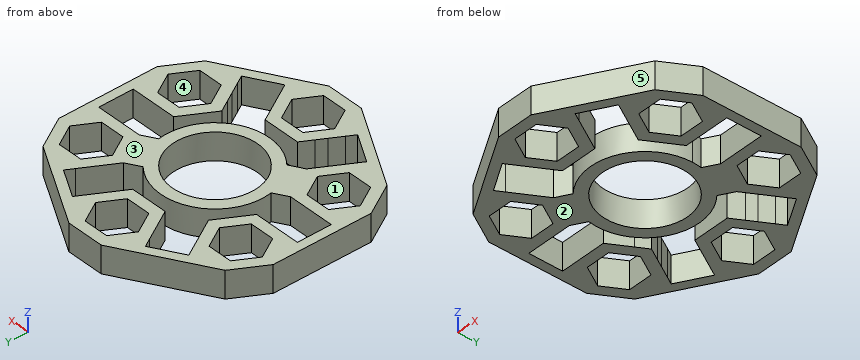
from build123d import *

# Parameters (mm, degrees)
F0_R     = 11.0786603321
F0_R_2   = 10.9474
F1_DEPTH = 6.9977
F2_R     = 13.2854455685
F2_R_2   = 11.176
F3_DEPTH = 6.9977


# Not quite as in the source:
# - a feature names something its author has since deleted; it is built from what else it names


with BuildPart() as f1:
    # F0 (on Top) → F1 (new body)
    with BuildSketch(Plane.XY):
        with BuildLine():
            ThreePointArc((8.9895158912, 10.693432753), (-6.985, 12.0983748909), (-13.7555423633, -2.438432753))
            ThreePointArc((-13.7555423633, -2.438432753), (-12.0983748909, -6.985), (-8.9895158912, -10.693432753))
            ThreePointArc((-8.9895158912, -10.693432753), (5.8981930708, -12.6638153216), (13.97, 0))
            ThreePointArc((13.97, 0), (13.9162823127, 1.2239226251), (13.7555423633, 2.438432753))
            ThreePointArc((13.7555423633, 2.438432753), (13.347336888, 4.1242572662), (12.7333664349, 5.7465014779))
            ThreePointArc((12.7333664349, 5.7465014779), (11.139521372, 8.4304189458), (8.9895158912, 10.693432753))
        make_face()
        Circle(F0_R, mode=Mode.SUBTRACT)
        Circle(F0_R)
        Circle(F0_R_2, mode=Mode.SUBTRACT)
        Polygon((-14.0807527651, 9.595996083), (-12.3768237899, 12.5472876405), (-14.2130055479, 15.7276477372), (-15.394837026, 17.7746399033), (-17.1428502621, 20.8022876405), (-21.9088767342, 20.8022876405), (-26.6749032064, 20.8022876405), (-31.4409296786, 12.5472876405), (-29.1460849644, 8.5725), (-26.6749032064, 4.2922876405), (-17.1428502621, 4.2922876405), (-15.3507527651, 7.3962915574), align=None)
        Polygon((-18.7559669142, 18.0082876405), (-15.6030570942, 12.5472876405), (-18.7559669142, 7.0862876405), (-25.0617865543, 7.0862876405), (-28.2146963743, 12.5472876405), (-25.0617865543, 18.0082876405), align=None, mode=Mode.SUBTRACT)
        Polygon((4.854194994, 33.5022876405), (-4.6778579503, 33.5022876405), (-7.0608711864, 29.3747876405), (-9.4438844224, 25.2472876405), (-4.6778579503, 16.9922876405), (-1.27, 16.9922876405), (1.27, 16.9922876405), (4.854194994, 16.9922876405), (6.6462924911, 20.0962915574), (7.9162924911, 22.295996083), (9.6202214662, 25.2472876405), (7.2372082301, 29.3747876405), align=None)
        Polygon((6.393988162, 25.2472876405), (3.2410783419, 19.7862876405), (-3.0647412982, 19.7862876405), (-6.2176511182, 25.2472876405), (-3.0647412982, 30.7082876405), (3.2410783419, 30.7082876405), align=None, mode=Mode.SUBTRACT)
        Polygon((-29.1460849644, -8.5725), (-31.5290982004, -12.7), (-26.7630717283, -20.955), (-21.9970452561, -20.955), (-17.231018784, -20.955), (-12.4649923118, -12.7), (-14.2130055479, -9.6723522628), (-15.4830055479, -7.4726477372), (-17.231018784, -4.445), (-20.7270452561, -4.445), (-23.2670452561, -4.445), (-26.7630717283, -4.445), align=None)
        Polygon((-25.150604473, -7.2393749809), (-18.8447848775, -7.2386250963), (-15.6912256606, -12.6992501153), (-18.8434860392, -18.1606250191), (-25.1493056347, -18.1613749037), (-28.3028648516, -12.7007498847), align=None, mode=Mode.SUBTRACT)
        Polygon((31.5290982004, 12.7), (26.7630717283, 20.955), (21.9970452561, 20.955), (17.231018784, 20.955), (12.4649923118, 12.7), (14.2130055479, 9.6723522628), (15.4830055479, 7.4726477372), (17.231018784, 4.445), (20.7270452561, 4.445), (23.2670452561, 4.445), (26.7630717283, 4.445), (29.1460849644, 8.5725), align=None)
        Polygon((25.1499550762, 7.239), (18.8441354361, 7.239), (15.691225616, 12.7), (18.8441354361, 18.161), (25.1499550762, 18.161), (28.3028648962, 12.7), align=None, mode=Mode.SUBTRACT)
        Polygon((-7.1490397082, -29.5275), (-4.7660264722, -33.655), (4.7660264722, -33.655), (7.1490397082, -29.5275), (9.5320529443, -25.4), (4.7660264722, -17.145), (1.27, -17.145), (-1.27, -17.145), (-4.7660264722, -17.145), (-6.5140397082, -20.1726477372), (-7.7840397082, -22.3723522628), (-9.5320529443, -25.4), align=None)
        Polygon((-6.3058196401, -25.4), (-3.15290982, -19.939), (3.15290982, -19.939), (6.3058196401, -25.4), (3.15290982, -30.861), (-3.15290982, -30.861), align=None, mode=Mode.SUBTRACT)
        Polygon((26.7630717283, -20.955), (31.5290982004, -12.7), (29.1460849644, -8.5725), (26.7630717283, -4.445), (17.231018784, -4.445), (12.4649923118, -12.7), (14.2130055479, -15.7276477372), (15.4830055479, -17.9273522628), (17.231018784, -20.955), (21.9970452561, -20.955), align=None)
        Polygon((18.8441354361, -18.161), (15.691225616, -12.7), (18.8441354361, -7.239), (25.1499550762, -7.239), (28.3028648962, -12.7), (25.1499550762, -18.161), align=None, mode=Mode.SUBTRACT)
        Polygon((-26.6749032064, 20.8022876405), (-21.9088767342, 20.8022876405), (-18.3343568801, 22.8660376405), (-10.6353910405, 27.3110376405), (-7.0608711864, 29.3747876405), (-4.6778579503, 33.5022876405), align=None)
        Polygon((-21.9970452561, -20.955), (-26.7630717283, -20.955), (-4.7660264722, -33.655), (-7.1490397082, -29.5275), (-10.7235595624, -27.46375), (-18.422525402, -23.01875), align=None)
        Polygon((31.5290982004, -12.7), (31.5290982004, 12.7), (29.1460849644, 8.5725), (29.1460849644, 4.445), (29.1460849644, -4.445), (29.1460849644, -8.5725), align=None)
        Polygon((7.1490397082, -29.5275), (4.7660264722, -33.655), (26.7630717283, -20.955), (21.9970452561, -20.955), (18.422525402, -23.01875), (10.7235595624, -27.46375), align=None)
        Polygon((26.7630717283, 20.955), (4.854194994, 33.5022876405), (7.2372082301, 29.3747876405), (10.811599772, 27.3357666355), (18.4011736203, 23.0062743808), (21.9970452561, 20.955), align=None)
        Polygon((-29.1460849644, 4.2922876405), (-29.1460849644, 8.5725), (-31.4409296786, 12.5472876405), (-31.5290982004, -12.7), (-29.1460849644, -8.5725), (-29.1460849644, -4.445), align=None)
        with BuildLine():
            Line((-13.7555423633, -2.438432753), (-17.231018784, -4.445))
            Line((-17.231018784, -4.445), (-15.4830055479, -7.4726477372))
            Line((-15.4830055479, -7.4726477372), (-14.2130055479, -9.6723522628))
            Line((-14.2130055479, -9.6723522628), (-12.4649923118, -12.7))
            Line((-12.4649923118, -12.7), (-8.9895158912, -10.693432753))
            ThreePointArc((-8.9895158912, -10.693432753), (-12.0983748909, -6.985), (-13.7555423633, -2.438432753))
        make_face()
        with BuildLine():
            Line((14.2130055479, 9.6723522628), (12.4649923118, 12.7))
            Line((12.4649923118, 12.7), (8.9895158912, 10.693432753))
            ThreePointArc((8.9895158912, 10.693432753), (11.139521372, 8.4304189458), (12.7333664349, 5.7465014779))
            ThreePointArc((12.7333664349, 5.7465014779), (13.347336888, 4.1242572662), (13.7555423633, 2.438432753))
            Line((13.7555423633, 2.438432753), (17.231018784, 4.445))
            Line((17.231018784, 4.445), (15.4830055479, 7.4726477372))
            Line((15.4830055479, 7.4726477372), (14.2130055479, 9.6723522628))
        make_face()
        Polygon((-29.1460849644, 4.2922876405), (-26.6749032064, 4.2922876405), (-29.1460849644, 8.5725), align=None)
        Polygon((10.811599772, 27.3357666355), (7.2372082301, 29.3747876405), (9.6202214662, 25.2472876405), align=None)
        Polygon((-21.9088767342, 20.8022876405), (-17.1428502621, 20.8022876405), (-18.3343568801, 22.8660376405), align=None)
        Polygon((-7.0608711864, 29.3747876405), (-10.6353910405, 27.3110376405), (-9.4438844224, 25.2472876405), align=None)
        Polygon((29.1460849644, 4.445), (29.1460849644, 8.5725), (26.7630717283, 4.445), align=None)
        Polygon((26.7630717283, -4.445), (29.1460849644, -8.5725), (29.1460849644, -4.445), align=None)
        Polygon((18.422525402, -23.01875), (21.9970452561, -20.955), (17.231018784, -20.955), align=None)
        Polygon((9.5320529443, -25.4), (7.1490397082, -29.5275), (10.7235595624, -27.46375), align=None)
        Polygon((-10.7235595624, -27.46375), (-7.1490397082, -29.5275), (-9.5320529443, -25.4), align=None)
        Polygon((-17.231018784, -20.955), (-21.9970452561, -20.955), (-18.422525402, -23.01875), align=None)
        Polygon((-26.7630717283, -4.445), (-29.1460849644, -4.445), (-29.1460849644, -8.5725), align=None)
        Polygon((17.231018784, 20.955), (21.9970452561, 20.955), (18.4011736203, 23.0062743808), align=None)
    extrude(amount=F1_DEPTH)

    # F2 (on Top) → F3 (join)
    with BuildSketch(Plane.XY):
        Circle(F2_R)
        Circle(F2_R_2, mode=Mode.SUBTRACT)
    extrude(amount=F3_DEPTH)


solid = f1.part
Build history of the part. All positions in model axes, mm. Face numbers are marked on the shaded views. A direction names the side the tool comes from. Round coordinates to 2 decimals unless told otherwise and drop trailing zeros. Write each loop counter-clockwise with the first axis right and the second up, starting at its lowest first coordinate (ties: lowest second). Pieces come first, ordered by that corner, then holes. Notation, with made-up numbers: M 88,54 L 121,54 A26 ccw 121,89 Z; hole C 80.5,28 d4. An arc over 180 degrees is marked long. Answer as a JSON object with one key per item and string values. Group by question number.
(1) Flat gauge pins, fed straight in: pin 1 (3 mm diameter, centred on x = -21.5, z = 4, fed in from +Y); pin 2 (1.5 mm diameter, centred on y = -0.5, z = 1.5, fed in from -X); pin 3 (1.5 mm diameter, centred on y = -20.5, z = 1.5, fed in from -X); pin 4 (1.5 mm diameter, centred on x = 5, y = -8, fed in from +Z). Where does each tip first touch, or does it go through?
(2) Mould opens along Y. For the marked faces 3, 4 and 5 say: pulls with the +Y half, pulls with the -Y half, needs draft (parallel to the pull), parting line crosses it, or undercut.
(3) Drill centre lines: L1, parallel to Y at x = 0, z = 2.25 (3 decimals); L2, parallel to Y at x = -15, z = 5.75; L3, parallel to X at y = -16, z = 6.75. Where is each one in solid material? Low to high.
(4) Which spindle directions (+Z, -Z, +X, -X, +Y, -Y) get a long thin tool onto all of the face, cutting with end or side? Do the marked faces 1 and 2. Say none if no direction does.
(5) Cut at B-B (z = 3.75). Give the number of separate pieces and of enclosed holes in the cut face, and give its area (3 significant figures).
(6) Cut at A-A (x = 0). Give the cut face in (y, z) (3 decimals), and give its area (3 significant figures).
Responses:
{
 "1": {"pin 1": "stops at y = 24.66", "pin 2": "stops at x = -31.49", "pin 3": "stops at x = -27.46", "pin 4": "passes through"},
 "2": {"face 3": "needs draft", "face 4": "undercut", "face 5": "pulls with the -Y half"},
 "3": {"L1": "y = -33.655 to -30.861, -19.939 to -17.145, -13.97 to -10.947, 10.947 to 13.97, 16.992 to 19.786, 30.708 to 33.502", "L2": "y = -27.75 to -24.99, -17.09 to -3.16, 8 to 17.09, 24.79 to 27.54", "L3": "x = -29.62 to -26.4, -17.6 to -14.37, 14.37 to 17.6, 26.4 to 29.62"},
 "4": {"face 1": "+Z, -Z", "face 2": "-Z, +X, -X, +Y, -Y"},
 "5": {"separate pieces": "1", "enclosed holes": "9", "area": "1,460 mm2"},
 "6": {"outline": "M -33.655,0 L -30.861,0 L -30.861,6.998 L -33.655,6.998 Z; M -19.939,0 L -17.145,0 L -17.145,6.998 L -19.939,6.998 Z; M -13.97,0 L -10.947,0 L -10.947,6.998 L -13.97,6.998 Z; M 10.947,0 L 13.97,0 L 13.97,6.998 L 10.947,6.998 Z; M 16.992,0 L 19.786,0 L 19.786,6.998 L 16.992,6.998 Z; M 30.708,0 L 33.502,0 L 33.502,6.998 L 30.708,6.998 Z", "area": "121 mm2"}
}
